Autodesk Inventor part; units mm, degrees
ref_plane "YZ Plane" through (0, 0, 0) normal (1, 0, 0) x (0, 1, 0)
ref_plane "XZ Plane" through (0, 0, 0) normal (0, 1, 0) x (-1, 0, 0)
sketch "Sketch1" plane through (0, 0, 0) normal (0, 1, 0) x (-1, 0, 0)
  line L0 (12.7, 114.3) -> (-12.7, 114.3)
  line L1 (-12.7, 114.3) -> (-12.7, -114.3)
  line L2 (-12.7, -114.3) -> (12.7, -114.3)
  line L3 (12.7, -114.3) -> (12.7, 114.3)
  line L4 (12.7, 114.3) -> (-12.7, -114.3) construction
  line L5 (-12.7, 114.3) -> (12.7, -114.3) construction
  point P0 (0, 0)
  dimension "d0" = 25.4
  dimension "d1" = 228.6
extrude "Extrusion1" add sketch "Sketch1" against normal blind 6.35
sketch "Sketch3" plane through (0, -6.35, 0) normal (0, -1, 0) x (1, 0, 0)
  circle A0 centre (0, 63.5) radius 6.35
  line L0 (12.7, 114.3) -> (-12.7, 114.3)
  point P0 (0, 0)
  dimension "d5" = 12.7
  dimension "d6" = 50.8
extrude "Extrusion2" cut sketch "Sketch3" against normal blind 3.556
sketch "Sketch4" plane through (0, -2.794, 63.5) normal (0, -1, 0) x (1, 0, 0)
  circle A0 centre (0, 0) radius 3.3782
  point P0 (0, -63.5)
  dimension "d9" = 6.7564
extrude "Extrusion3" cut sketch "Sketch4" against normal through all
ref_plane "Work Plane2" through (-12.7, 0, 76.2) normal (0, 0, 1) x (1, 0, 0)
mirror "Mirror1" about plane through (-12.7, 0, 76.2) normal (0, 0, 1) of "Extrusion3", "Extrusion2"
mirror "Mirror2" about plane through (0, 0, 0) normal (0, 0, 1) of "Extrusion3", "Extrusion2", "Mirror1"
properties part number "BandSawJigSupport"
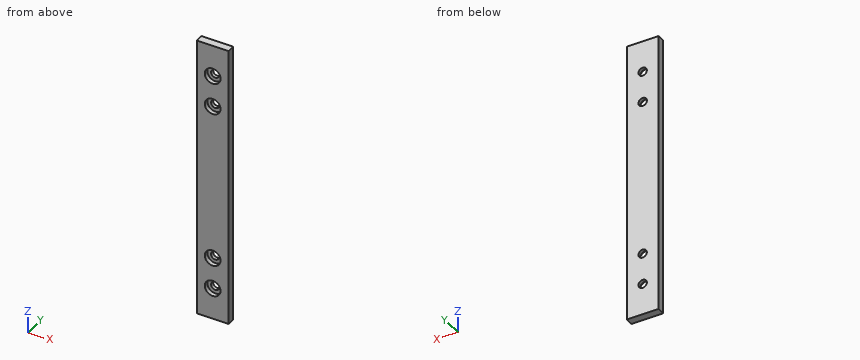
The listing builds one solid part. Answer for the finished solid, in the listing's coordinates (mm). Round coordinates to 2 decimals unless told otherwise and drop trailing zeros. Order: outer loops, then holes, each group sorted by start corner. A loop starts at its lowest first (then second) coordinate and runs counter-clockwise, first axis right, second up. Notation, with made-up numbers: M -29,48 L 11,48 A20 ccw 11,78 Z; hole C -33.5,54.5 d9. An arc over 180 degrees is marked long. Answer in a Markdown table with one row per item. Add a question column.
1) A flat-ended cylindrical pin translates along its axis: pin 1 Ø10 at (x, z) = (0, 88.9) entering from -Y. Find the tip coordinate at first contact, or state that the pin passes through.
2) The part is cut by section C-C on x = 0. Count the separate pieces of the cut face and the enclosed holes in it, plus the area to 3 significant figures.
3) The part is cut by section B-B on y = -3.75. Determine the outline of the cut face in (x, z), plus the area to 3 significant figures.
4) Consider line 1 along Z through (x, y) = (0, -3.85); line 2 along Z through (x, y) = (0, -2.05); line 3 along X through (y, z) = (-1.1, 88.9). Determine where each line is inside the solid, lowest interval first. Write a range as from..to.
5) The part is cut by section A-A on z = -63.5. Determine the outline of the cut face in (x, y), plus the area to 3 significant figures.
Findings below:
| question | item | result |
|---|---|---|
| 1 | pin 1 | stops at y = -2.79 |
| 2 | separate pieces | 5 |
| 2 | enclosed holes | 0 |
| 2 | area | 1,200 mm² |
| 3 | outline | M -12.7,-114.3 L 12.7,-114.3 L 12.7,114.3 L -12.7,114.3 Z; hole C 0,-88.9 d12.7; hole C 0,-63.5 d12.7; hole C 0,63.5 d12.7; hole C 0,88.9 d12.7 |
| 3 | area | 5,300 mm² |
| 4 | line 1 | z = -114.3..-95.25, -82.55..-69.85, -57.15..57.15, 69.85..82.55, 95.25..114.3 |
| 4 | line 2 | z = -114.3..-92.28, -85.52..-66.88, -60.12..60.12, 66.88..85.52, 92.28..114.3 |
| 4 | line 3 | x = -12.7..-3.38, 3.38..12.7 |
| 5 | outline | M -12.7,-6.35 L -6.35,-6.35 L -6.35,-2.79 L -3.38,-2.79 L -3.38,0 L -12.7,0 Z; M 3.38,-2.79 L 6.35,-2.79 L 6.35,-6.35 L 12.7,-6.35 L 12.7,0 L 3.38,0 Z |
| 5 | area | 97.3 mm² |
